```python
from build123d import *

# Parameters (mm, degrees)
SCHIZZO1_W                   = 140.36
SCHIZZO1_H                   = 280
ESTRUSIONE_ESTRUSIONE1_DEPTH = 3
SCHIZZO2_R                   = 2
TAGLIO_ESTRUSIONE1_DEPTH     = 4
SCHIZZO3_W                   = 45
SCHIZZO3_H                   = 45
TAGLIO_ESTRUSIONE2_DEPTH     = 4
SCHIZZO4_R                   = 1.5
SCHIZZO4_R_2                 = 2
TAGLIO_ESTRUSIONE3_DEPTH     = 4


with BuildPart() as part:
    # Schizzo1 → Estrusione-Estrusione1 (new body)
    with BuildSketch(Plane(origin=(0, 0, 0), x_dir=(1, 0, 0), z_dir=(0, 1, 0))):
        with Locations((-26.670393701, -27.952755906)):
            Rectangle(SCHIZZO1_W, SCHIZZO1_H)
    extrude(amount=ESTRUSIONE_ESTRUSIONE1_DEPTH)

    # Schizzo2 → Taglio-Estrusione1 (cut, through all)
    with BuildSketch(Plane(origin=(0, 3, 0), x_dir=(1, 0, 0), z_dir=(0, 1, 0))):
        with Locations((-86.850393701, -152.952755906)):
            Circle(SCHIZZO2_R)
        with Locations((33.509606299, -152.952755906)):
            Circle(SCHIZZO2_R)
        with Locations((-86.850393701, 97.047244094)):
            Circle(SCHIZZO2_R)
        with Locations((33.509606299, 97.047244094)):
            Circle(SCHIZZO2_R)
    extrude(amount=-TAGLIO_ESTRUSIONE1_DEPTH, mode=Mode.SUBTRACT)

    # Schizzo3 → Taglio-Estrusione2 (cut, through all)
    with BuildSketch(Plane(origin=(0, 0, 0), x_dir=(1, 0, 0), z_dir=(0, 1, 0))):
        with Locations((-74.350393701, -69.752755906)):
            Rectangle(SCHIZZO3_W, SCHIZZO3_H)
        with Locations((21.009606299, -69.752755906)):
            Rectangle(SCHIZZO3_W, SCHIZZO3_H)
    extrude(amount=TAGLIO_ESTRUSIONE2_DEPTH, mode=Mode.SUBTRACT)

    # Schizzo4 → Taglio-Estrusione3 (cut, through all)
    with BuildSketch(Plane(origin=(0, 0, 0), x_dir=(1, 0, 0), z_dir=(0, 1, 0))):
        with Locations((-85.170393701, 87.047244094)):
            Circle(SCHIZZO4_R)
        with Locations((-85.170393701, -29.952755906)):
            Circle(SCHIZZO4_R)
        with Locations((31.829606299, -29.952755906)):
            Circle(SCHIZZO4_R)
        with Locations((31.829606299, 87.047244094)):
            Circle(SCHIZZO4_R)
        with Locations((-43.180393701, -89.952755906)):
            Circle(SCHIZZO4_R)
        with Locations((-10.160393701, -89.952755906)):
            Circle(SCHIZZO4_R)
        with Locations((-10.160393701, -122.972755906)):
            Circle(SCHIZZO4_R)
        with Locations((-43.180393701, -122.972755906)):
            Circle(SCHIZZO4_R)
        with Locations((-52.470393701, -97.952755906)):
            Circle(SCHIZZO4_R_2)
        with Locations((-0.870393701, -97.952755906)):
            Circle(SCHIZZO4_R_2)
        with Locations((-0.870393701, 32.647244094)):
            Circle(SCHIZZO4_R_2)
        with Locations((-52.470393701, 32.647244094)):
            Circle(SCHIZZO4_R_2)
        with Locations((-74.295393701, -124.312755906)):
            Circle(SCHIZZO4_R)
        with Locations((20.954606299, -124.312755906)):
            Circle(SCHIZZO4_R)
        with Locations((20.954606299, -164.952755906)):
            Circle(SCHIZZO4_R)
        with Locations((-74.295393701, -164.952755906)):
            Circle(SCHIZZO4_R)
    extrude(amount=TAGLIO_ESTRUSIONE3_DEPTH, mode=Mode.SUBTRACT)


solid = part.part
```
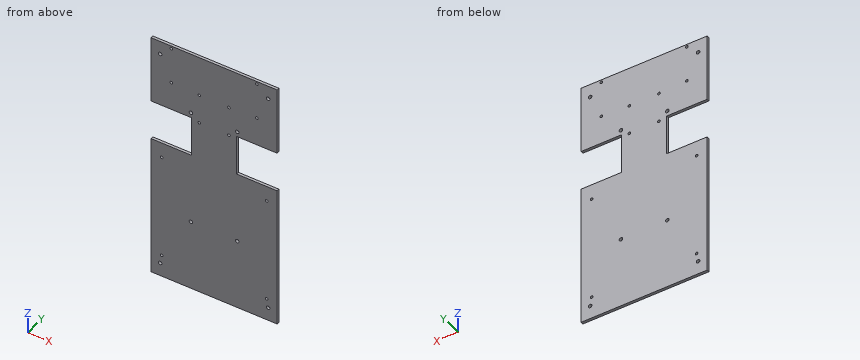
Geometry: final body of the model. Coordinates: model frame, mm. Round coordinates to 2 decimals unless told otherwise and drop trailing zeros. Order: outer loops, then holes, each group sorted by start corner. A loop starts at its lowest first (then second) coordinate and runs counter-clockwise, first axis right, second up. Notation, with made-up numbers: (87, -38.75) - (146, -38.75) arc R25 ccw to (146, -4.75) - close; hole circle Ø9 at (58.25, -15.75). An arc over 180 degrees is marked (long way). Write item = value, one per line. Start each with the question number.
Q1. Cut plane C-C on z = 85.5. Return the cut outline in (x, y).
Q2. Pin query (flat end, axial travel): pin 1 (3.5 mm diameter, centred on x = -0.87, z = 97.95, fed in from +Y). Return the tip coordinate at first contact, or that it passes through.
Q3. Cut plane B-B on y = 1.35. Give the number of separate pieces and of enclosed holes in the cut face, and give its area (3 significant figures).
Q4. Cut plane A-A on x = -79.5. Return the cut outline in (y, z), and give its area (3 significant figures).
Q5. Ray query, line 1 (Z direction, x = 21, y = 2.65); line 2 (Z direction, x = 30, y = 2.1); line 3 (Z direction, x = -53.5, y = 1.7). Return the intervals inside material, ascending. Write a range as from..to.
Outcome:
q1.outline = (-51.85, 0) - (-1.49, 0) - (-1.49, 3) - (-51.85, 3) - close
q2.pin_1 = through
q3.separate_pieces = 1
q3.enclosed_holes = 20
q3.area = 35,100 mm^2
q4.outline = (0, -112.05) - (3, -112.05) - (3, 47.25) - (0, 47.25) - close; (0, 92.25) - (3, 92.25) - (3, 167.95) - (0, 167.95) - close
q4.area = 705 mm^2
q5.line_1 = -112.05..47.25, 92.25..122.81, 125.81..163.45, 166.45..167.95
q5.line_2 = -112.05..47.25, 92.25..167.95
q5.line_3 = -112.05..-34.36, -30.93..47.25, 92.25..96.24, 99.67..167.95
